from build123d import *

# Parameters (mm, degrees)
SKETCH1_W           = 31.75
SKETCH1_H           = 31.75
SKETCH1_W_2         = 24.13
SKETCH1_H_2         = 24.13
BOSS_EXTRUDE1_DEPTH = 762
SKETCH14_W          = 31.75
SKETCH14_H          = 31.75
SKETCH14_W_2        = 25.4
SKETCH14_H_2        = 25.4
BOSS_EXTRUDE2_DEPTH = 685.8
SKETCH14_2_W        = 25.4
SKETCH14_2_H        = 25.4
BOSS_EXTRUDE3_DEPTH = 2.54
BOSS_EXTRUDE6_START = -683.26
SKETCH14_3_W        = 25.4
SKETCH14_3_H        = 25.4
BOSS_EXTRUDE6_DEPTH = 2.54
SKETCH1_2_W         = 24.13
SKETCH1_2_H         = 24.13
BOSS_EXTRUDE4_DEPTH = 2.54
BOSS_EXTRUDE5_START = 759.46
SKETCH1_3_W         = 24.13
SKETCH1_3_H         = 24.13
BOSS_EXTRUDE5_DEPTH = 2.54
LPATTERN4_COUNT     = 3
LPATTERN4_PITCH     = 365.125


with BuildPart() as part:
    # Sketch1 → Boss-Extrude1 (new body)
    with BuildSketch(Plane.XY):
        Rectangle(SKETCH1_W, SKETCH1_H)
        Rectangle(SKETCH1_W_2, SKETCH1_H_2, mode=Mode.SUBTRACT)
    extrude(amount=BOSS_EXTRUDE1_DEPTH)

    # Sketch14 → Boss-Extrude2 (add)
    with BuildSketch(Plane.XZ.offset(15.875)):
        with Locations((0, 746.125)):
            Rectangle(SKETCH14_W, SKETCH14_H)
        with Locations((0, 746.125)):
            Rectangle(SKETCH14_W_2, SKETCH14_H_2, mode=Mode.SUBTRACT)
    boss_extrude2 = extrude(amount=-BOSS_EXTRUDE2_DEPTH)

    # Sketch14<2> → Boss-Extrude3 (add)
    with BuildSketch(Plane.XZ.offset(15.875)):
        with Locations((0, 746.125)):
            Rectangle(SKETCH14_2_W, SKETCH14_2_H)
    boss_extrude3 = extrude(amount=-BOSS_EXTRUDE3_DEPTH)

    # Sketch14<3> → Boss-Extrude6 (add)
    with BuildSketch(Plane.XZ.offset(15.875).offset(BOSS_EXTRUDE6_START)):
        with Locations((0, 746.125)):
            Rectangle(SKETCH14_3_W, SKETCH14_3_H)
    boss_extrude6 = extrude(amount=-BOSS_EXTRUDE6_DEPTH)

    # Sketch1<2> → Boss-Extrude4 (add)
    with BuildSketch(Plane.XY):
        Rectangle(SKETCH1_2_W, SKETCH1_2_H)
    extrude(amount=BOSS_EXTRUDE4_DEPTH)

    # Sketch1<3> → Boss-Extrude5 (add)
    with BuildSketch(Plane.XY.offset(BOSS_EXTRUDE5_START)):
        Rectangle(SKETCH1_3_W, SKETCH1_3_H)
    extrude(amount=BOSS_EXTRUDE5_DEPTH)

    # LPattern4: Boss-Extrude2, Boss-Extrude3, Boss-Extrude6 ×3
    with Locations(*[(0, 0, -i * LPATTERN4_PITCH) for i in range(1, LPATTERN4_COUNT)]):
        add(boss_extrude2)
        add(boss_extrude3)
        add(boss_extrude6)


solid = part.part
Source: CAD feature listing. Evaluate the final solid. Frame: model axes, mm. A direction names the side the tool comes from. Coordinates: 2 decimals unless noted, no trailing zeros. Loops run counter-clockwise (first coordinate to the right, second up) from the corner with the lowest first, then second, coordinate; pieces in that order, holes last. Notation, with made-up numbers: (-10.5, -31.5) - (1.5, -31.5) arc R14 ccw to (1.5, -7.5) - close; hole circle Ø2 at (51.5, 53). An arc over 180 degrees is marked (long way). Return JSON: item names as keys, results as strings.
Q1. Section B-B, the plane z = 634.5. Return loops of the section in (x, y) (3 decimals), plus the area to 3 significant figures.
Results:
{"outline": "(-15.875, -15.875) - (15.875, -15.875) - (15.875, 15.875) - (-15.875, 15.875) - close; hole (-12.065, -12.065) - (12.065, -12.065) - (12.065, 12.065) - (-12.065, 12.065) - close", "area": "426 mm2"}
Q2. Section C-C, the plane x = 0. Give the number of separate pieces and of enclosed holes in the cut face, plus the area to 3 significant figures.
Results:
{"separate pieces": "1", "enclosed holes": "8", "area": "18,900 mm2"}
Q3. Material intervals for line 1 along Z through (x, y) = (-9.5, 477) (3 decimals); line 2 along Y through (x, z) = (-10.5, 372) (3 decimals); line 3 along Z through (x, y) = (-13, 72) (3 decimals), sorted ascending.
Results:
{"line 1": "0 to 3.175, 28.575 to 31.75, 365.125 to 368.3, 393.7 to 396.875, 730.25 to 733.425, 758.825 to 762", "line 2": "-15.875 to -12.065, 12.065 to 15.875, 667.385 to 669.925", "line 3": "0 to 31.75, 365.125 to 396.875, 730.25 to 762"}
Q4. Access query for faces 4 (the flat face through (0, 669.925, 381)), 5 (the flat face through (12.065, 0, 16)), 6 (the flat face through (0, 338, 31.75)). Directions: +Z, -Z, +X, -X, +Y, -Y. A direction counts if a zero-diameter tool reaches every point of the face in a straight line with its end or side. Return the directions, or none.
Results:
{"face 4": "+Z, -Z, +X, -X, +Y", "face 5": "none", "face 6": "+X, -X, +Y"}
Q5. Section A-A, the plane y = 233. Return loops of the section in (x, z) (3 decimals).
Results:
{"outline": "(-15.875, 0) - (15.875, 0) - (15.875, 31.75) - (-15.875, 31.75) - close; (-15.875, 365.125) - (15.875, 365.125) - (15.875, 396.875) - (-15.875, 396.875) - close; (-15.875, 730.25) - (15.875, 730.25) - (15.875, 762) - (-15.875, 762) - close; hole (-12.7, 3.175) - (12.7, 3.175) - (12.7, 28.575) - (-12.7, 28.575) - close; hole (-12.7, 368.3) - (12.7, 368.3) - (12.7, 393.7) - (-12.7, 393.7) - close; hole (-12.7, 733.425) - (12.7, 733.425) - (12.7, 758.825) - (-12.7, 758.825) - close"}
Q6. Mould query, pull axis Z, two halves, no side actions, for faces 1 (the flat face through (0, -12.065, 746)), 2 (the flat face through (0, 669.925, 746)), 3 (the flat face through (0, 332, 0)). Classes: released by +Z, released by -Z, zero draft, split by the parting line, or undercut.
Results:
{"face 1": "undercut", "face 2": "zero draft", "face 3": "released by -Z"}
